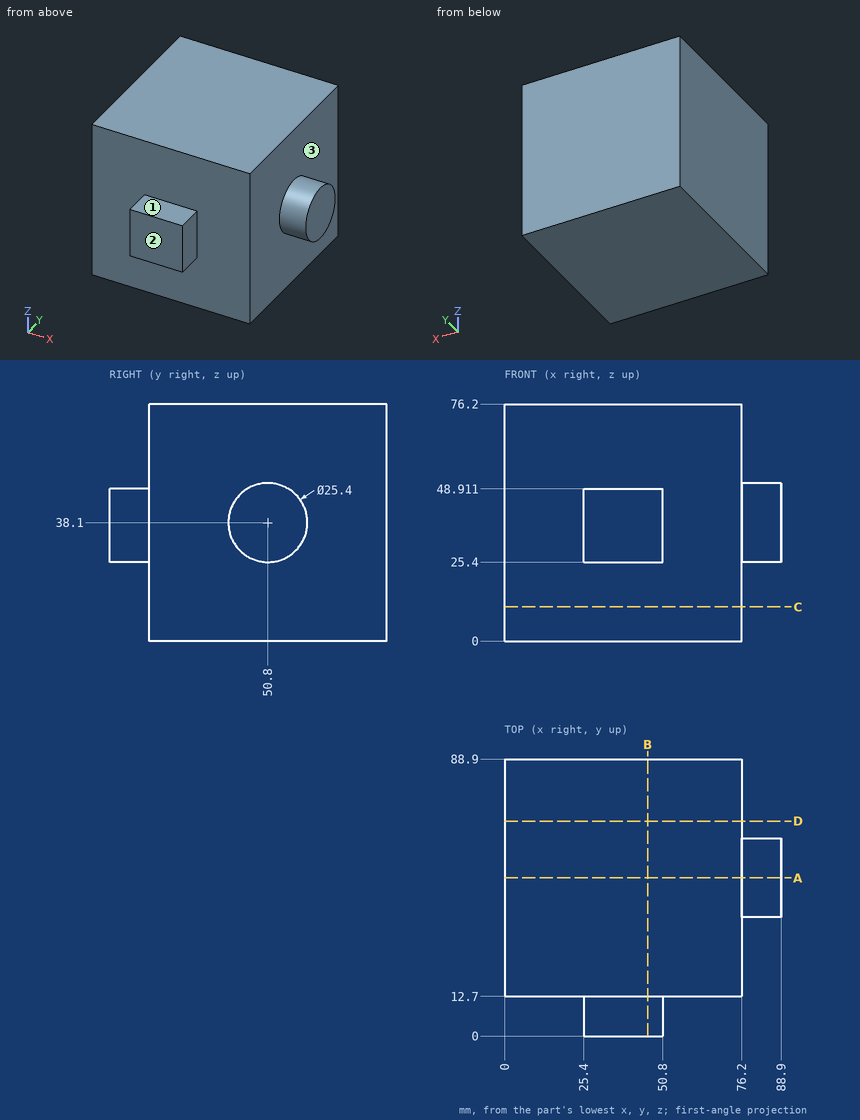
Source: three-view drawing plus pictorial views. Frame: mm from the lowest corner of the part. A direction names the side the tool comes from. Give positions to 0.01 mm unless a question says otherwise; leave off trailing zeros. Order: outer loops, then holes, each group sorted by start corner. A loop starts at its lowest first (then second) coordinate and runs counter-clockwise, first axis right, second up. Notation, with made-up numbers: M -28,11 L -17,11 A28 cw -17,41 Z; hole C -32.75,-32.75 d3. An arc over 180 degrees is marked long. One line per question, with ' | ' between items. Start each with the question number.
1. Section query D-D (y = 69). Return the cut outline in (x, z).
2. Section query A-A (y = 50.8). Return the cut outline in (x, z), and give its area (3 significant figures).
3. Material intervals for probe 1 along Y at (x, z) = (44, 63.5); probe 2 along X at (y, z) = (76, 47); probe 3 along X at (y, z) = (4.5, 32.5), sorted ascending. Write a range as [from, to].
4. Section query B-B (x = 46). Return the cut outline in (y, z).
5. Section query C-C (z = 11). Return the cut outline in (x, y).
6. First-contact query: pin 1 Ø14 at (x, y) = (34.5, 5) entering from +Z; pin 2 Ø6.5 at (y, z) = (6, 36.5) entering from +X; pin 3 Ø10 at (y, z) = (26, 17) entering from +X. Flat tips, straight axial feed; report the tip coordinate or a pass-through.
7. Access query for the marked faces 1, 2 and 3. Directions: +Z, -Z, +X, -X, +Y, -Y. A direction counts if a zero-diameter tool reaches every point of the face in a straight line with its end or side. Return the directions, or none.
Here are the results:
1) outline: M 0,0 L 76.2,0 L 76.2,76.2 L 0,76.2 Z
2) outline: M 0,0 L 76.2,0 L 76.2,25.4 L 88.9,25.4 L 88.9,50.8 L 76.2,50.8 L 76.2,76.2 L 0,76.2 Z | area: 6,130 mm²
3) probe 1: [12.7, 88.9] | probe 2: [0, 76.2] | probe 3: [25.4, 50.8]
4) outline: M 0,25.4 L 12.7,25.4 L 12.7,0 L 88.9,0 L 88.9,76.2 L 12.7,76.2 L 12.7,48.91 L 0,48.91 Z
5) outline: M 0,12.7 L 76.2,12.7 L 76.2,88.9 L 0,88.9 Z
6) pin 1: z = 48.91 | pin 2: x = 50.8 | pin 3: x = 76.2
7) face 1: +Z, +X, -X, -Y | face 2: +Z, -Z, +X, -X, -Y | face 3: +X
